Autodesk Inventor part; units mm, degrees
ref_plane "Work Plane2" through (-135, -43.5, 18) normal (0, 0, -1) x (0, 1, 0)
ref_plane "YZ Plane" through (0, 0, 0) normal (1, 0, 0) x (0, 1, 0)
ref_plane "XZ Plane" through (0, 0, 0) normal (0, 1, 0) x (-1, 0, 0)
ref_plane "Work Plane1" through (0, 0, 0) normal (0, 0, 1) x (1, 0, 0)
sketch "Sketch1" plane through (0, 0, 0) normal (0, 0, 1) x (1, 0, 0)
  circle A0 centre (119.5, 7) radius 3.3
  circle A1 centre (119.5, 38) radius 3.3
  circle A2 centre (88.5, 38) radius 3.3
  circle A3 centre (88.5, 7) radius 3.3
  circle A4 centre (104, 22.5) radius 11
  circle A5 centre (-76, 8.5) radius 1.7
  circle A6 centre (-76, 38) radius 1.7
  circle A7 centre (-45, -33.5) radius 4.3
  circle A8 centre (-45, -3) radius 4.3
  circle A9 centre (-60.5, 12.5) radius 1.7
  circle A10 centre (-60.5, 43.5) radius 1.7
  circle A11 centre (-29.5, 43.5) radius 1.7
  circle A12 centre (-29.5, 12.5) radius 1.7
  circle A13 centre (-45, 28) radius 11.5
  circle A14 centre (-122.5, -32.5) radius 3.3
  circle A15 centre (-83.5, -32.5) radius 3.3
  circle A16 centre (83.5, -32.5) radius 3.3
  circle A17 centre (122.5, -32.5) radius 3.3
  circle A18 centre (-103, 22.5) radius 2.75
  circle A19 centre (78, 8.5) radius 1.7
  circle A20 centre (78, 38) radius 1.7
  circle A21 centre (-130, 8.5) radius 1.7
  circle A22 centre (-130, 38) radius 1.7
  circle A23 centre (130, 38) radius 1.7
  circle A24 centre (130, 8.5) radius 1.7
  arc A25 (-135, -38.5) -> (-130, -43.5) centre (-130, -38.5) ccw
  line L0 (130, -43.5) -> (-130, -43.5)
  arc A26 (130, -43.5) -> (135, -38.5) centre (130, -38.5) ccw
  line L1 (135, 38.5) -> (135, -38.5)
  arc A27 (135, 38.5) -> (130, 43.5) centre (130, 38.5) ccw
  line L2 (-24, 43.5) -> (130, 43.5)
  line L3 (-24, 43.5) -> (-24, 45.5)
  line L4 (-24, 45.5) -> (-27.5, 49)
  line L5 (-27.5, 49) -> (-62.5, 49)
  line L6 (-62.5, 49) -> (-66, 45.5)
  line L7 (-66, 45.5) -> (-66, 43.5)
  line L8 (-130, 43.5) -> (-66, 43.5)
  arc A28 (-130, 43.5) -> (-135, 38.5) centre (-130, 38.5) ccw
  line L9 (-135, -38.5) -> (-135, 38.5)
  line L10 (-115.5, -26.5) -> (-115.5, -38.5)
  line L11 (-90.5, -26.5) -> (-115.5, -26.5)
  line L12 (-90.5, -38.5) -> (-90.5, -26.5)
  line L13 (-115.5, -38.5) -> (-90.5, -38.5)
  line L14 (117.5, -38.5) -> (117.5, -26.5)
  line L15 (90.5, -38.5) -> (117.5, -38.5)
  line L16 (90.5, -26.5) -> (90.5, -38.5)
  line L17 (117.5, -26.5) -> (90.5, -26.5)
  line L18 (130, 38) -> (130, 8.5) construction
  line L19 (127.3, 38) -> (127.3, 8.5)
  arc A29 (130, 40.7) -> (127.3, 38) centre (130, 38) ccw
  arc A30 (127.3, 8.5) -> (130, 5.8) centre (130, 8.5) ccw
  line L20 (135, 38.5) -> (135, 40.7)
  line L21 (130, 5.8) -> (138.5, 5.8)
  line L22 (135.5, 40.7) -> (135.5, 5.8)
  line L23 (138.5, 40.7) -> (138.5, 5.8)
  line L24 (138.5, 40.7) -> (130, 40.7)
  point P0 (0, 0)
  point P1 (130, 23.25)
  dimension "d0" = 5.4
  dimension "d1" = 0.5
  dimension "d2" = 3
ref_plane "Work Plane2" through (-135, -43.5, 18) normal (0, 0, -1) x (0, 1, 0)
extrude "Extrusion1" add sketch "Sketch1" along normal up to surface (18 mm away) contours A23 | A24 | L21 A30 L19 A29 L24 A27 L1 | L1 L20 L24 L22 L21 | A27 L24 L20 | L22 L24 L23 L21
sketch "Sketch2" plane through (130, 40.7, 18) normal (0, 0, 1) x (1, 0, 0)
  arc A0 (0, 0) -> (-2.7, -2.7) centre (0, -2.7) ccw
  line L0 (8.5, 0) -> (0, 0)
  line L1 (8.5, -34.9) -> (8.5, 0)
  line L2 (0, -34.9) -> (8.5, -34.9)
  arc A1 (-2.7, -32.2) -> (0, -34.9) centre (0, -32.2) ccw
  line L3 (-2.7, -2.7) -> (-2.7, -32.2)
  line L4 (5.5, 0) -> (5.5, -34.9)
  line L5 (5, -2.2) -> (5, 0)
  line L6 (5, -2.2) -> (5, -79.2)
  point P0 (-130, -40.7)
extrude "Extrusion2" add sketch "Sketch2" along normal blind 18 contours L0 L1 L2 L4
sketch "Sketch3" plane through (138.5, 5.8, 0) normal (1, 0, 0) x (0, 0, -1)
  line L0 (-36, 0) -> (-36, 34.9)
  line L1 (-22, 32.7) -> (-22, -44.3)
  line L2 (-22, 32.7) -> (-22, 37.7)
  circle A0 centre (-29, 17.45) radius 7.5
  line L3 (-36, 17.45) -> (-22, 17.45) construction
  line L4 (-18, 37.7) -> (-18, 32.7)
  line L5 (-18, 32.7) -> (-18, -44.3)
  line L6 (-18, 34.9) -> (-36, 34.9)
  line L7 (0, 0) -> (-36, 0)
  line L8 (-18, 34.9) -> (-33.4562, 23.4826)
  line L9 (-33.4562, 11.4174) -> (-18, 0)
  circle A1 centre (-29, 17.45) radius 6
  point P0 (0, -5.8)
  point P1 (-36, 20.1426)
  point P2 (-36, 14.7574)
  point P3 (-22, 20.1426)
  point P4 (-22, 14.7574)
  dimension "d7" = 15
  dimension "d8" = 12
extrude "Extrusion3" cut sketch "Sketch3" against normal through all contours L0 A0 L9 L1 L7 | A0 L0 | L1 L9 L7 | L0 L6 L2 L1 L8 A0 | L6 L8 L1 L2 | A1
properties part number "tumbler_holdeerr"
The listing builds one solid part. Answer for the finished solid, in the listing's coordinates (mm). A direction names the side the tool comes from. Coordinates: 2 decimals unless noted, no trailing zeros. Write each loop counter-clockwise with the first axis right and the second up, starting at its lowest first coordinate (ties: lowest second). Pieces come first, ordered by that corner, then holes. Notation, with made-up numbers: M 23.25,-12 L 60.25,-12 A25 cw 60.25,19 Z; hole C -33.75,8.25 d4. An arc over 180 degrees is marked long. Put each result on its own line as item: value. Start each with the question number.
1. Which of the six approach directions +Z, -Z, +X, -X, +Y, -Y give full straight-line access (tool end or side, diameter ignored) to faces 1 (the flat face through (131, 23, 18)), 2 (the cylindrical face through (128.11, 6.57, 8.87))?
2. Flat-ended cylindrical pins translate along their axes: P1, Ø1.5, axis at x = 131, z = 20.5, coming from the +Y side; P2, Ø5.5, axis at y = 20.5, z = 23, coming from the -X side. Find the tip coordinate at first contact, or state that the pin passes through.
3. Consider line 1 (X direction, y = 31, z = 30.5); line 2 (Z direction, x = 135.25, y = 17); line 3 (Y direction, x = 137, z = 29). Determine where each line is inside the solid, lowest interval first. Write a range as from..to.
4. A cutting plane is placed at A-A on y = 23.25. Write down the section's boundary in (x, z).
5. A cutting plane is placed at B-B on x = 137. Write down the section's boundary in (y, z).
6. A cutting plane is placed at D-D on y = 30. Write down the section's boundary in (x, z), then the cut area to 3 significant figures.
7. A cutting plane is placed at C-C on z = 23.5. Write down the section's boundary in (x, y), then the cut area to 3 significant figures.
8. For a pull along Y with two mould halves and no side action, classify faces 3 (the flat face through (135.5, 23, 21)), 4 (the flat face through (134, 40.7, 9)), 5 (the cylindrical face through (137.021, 23.514, 34.994)), 6 (the cylindrical face through (137.021, 18.73, 34.985)) as pulls with the +Y half, pulls with the -Y half, needs draft (parallel to the pull), parting line crosses it, or undercut.
Resolved:
1. face 1: +Z, -X, +Y, -Y
1. face 2: +Z, -Z, -X, -Y
2. P1: passes through
2. P2: stops at x = 135.5
3. line 1: x = 135.5..138.5
3. line 2: z = 0..18
3. line 3: y = 13.93..17.25, 29.25..32.57
4. outline: M 127.3,0 L 138.5,0 L 138.5,23 L 135.5,23 L 135.5,18 L 127.3,18 Z; M 135.5,35 L 138.5,35 L 138.5,36 L 135.5,36 Z
5. outline: M 5.8,0 L 40.7,0 L 40.7,18 L 29.28,33.46 A7.5 ccw 25.94,36 L 20.56,36 A7.5 ccw 17.22,33.46 L 5.8,18 Z; hole C 23.25,29 d12
6. outline: M 127.3,0 L 138.5,0 L 138.5,32.49 L 135.5,32.49 L 135.5,18 L 127.3,18 Z
6. area: 245 mm2
7. outline: M 135.5,9.86 L 138.5,9.86 L 138.5,20.85 L 135.5,20.85 Z; M 135.5,25.65 L 138.5,25.65 L 138.5,36.64 L 135.5,36.64 Z
7. area: 65.9 mm2
8. face 3: needs draft
8. face 4: pulls with the +Y half
8. face 5: undercut
8. face 6: pulls with the -Y half
